CAD build for the part. Positions are in the model's coordinates, mm. Coordinates: 2 decimals unless noted, no trailing zeros. Loops run counter-clockwise (first coordinate to the right, second up) from the corner with the lowest first, then second, coordinate; pieces in that order, holes last. Notation, with made-up numbers: (4, -37.75) -> (10, -37.75) arc R17 cw to (10, -8.75) -> close; hole circle Ø7 at (35, -26). An arc over 180 degrees is marked (long way). Answer as a JSON object with one key per item and string values. Group by question number.
from build123d import *

# Parameters (mm, degrees)
SKETCH1_R           = 10
BOSS_EXTRUDE1_DEPTH = 60


with BuildPart() as part:
    # Sketch1 → Boss-Extrude1 (new body)
    with BuildSketch(Plane.XY):
        with BuildLine():
            Line((0, 0), (60, 0))
            Line((60, 0), (60, 60))
            ThreePointArc((60, 60), (30, 90), (0, 60))
            Line((0, 60), (0, 0))
        make_face()
        with Locations((30, 60)):
            Circle(SKETCH1_R, mode=Mode.SUBTRACT)
    extrude(amount=BOSS_EXTRUDE1_DEPTH)

    # Sketch4 → Cut-Revolve1 (revolve, cut)
    with BuildSketch(Plane.XY.offset(30)):
        with BuildLine():
            Line((30, 30), (30, -10))
            ThreePointArc((30, -10), (50, 10), (30, 30))
        make_face()
    revolve(axis=Axis((30, 30, 30), (0, -1, 0)), mode=Mode.SUBTRACT)


solid = part.part
Item 1: Band-saw the part on A-A, the plane z = 18. List the corners of the cut face in (x, y), and give its area (3 significant figures).
Item 2: Flat gauge pins, fed straight in: P1, Ø1, axis at y = 64.5, z = 48.5, coming from the -X side; P2, Ø2, axis at y = 64, z = 8.5, coming from the -X side. Where does each tip first touch, or does it go through?
Item 3: Pull direction Y, two halves, no side cores. Call faces 1 (the cylindrical face through (39.237, 56.17, 29.58)), 2 (the flat face through (30, 46, 60)), 3 (the cylindrical face through (30.66, 89.993, 29.58)): +Y half, -Y half, draft (parallel to the pull), parting line (faces both ways), or undercut.
Item 4: Drill centre lines: L1, parallel to Y at x = 30, z = 30; L2, parallel to X at y = 59.5, z = 5; L3, parallel to X at y = 66, z = 10. Where is each one in solid material? Low to high.
Item 5: Band-saw the part on C-C, the plane x = 30. List the corners of the cut face in (y, z).
Item 6: Band-saw the part on D-D, the plane y = 9. List the corners of the cut face in (x, z).
Item 7: Band-saw the part on B-B, the plane y = 55. List the corners of the cut face in (x, z).
Reply:
{
 "1": {"outline": "(0, 0) -> (17.51, 0) arc R16 cw (long way) to (42.49, 0) -> (60, 0) -> (60, 60) arc R30 ccw to (0, 60) -> close; hole circle Ø20 at (30, 60)", "area": "4,000 mm²"},
 "2": {"P1": "x = 0.27", "P2": "x = 0.15"},
 "3": {"face 1": "undercut", "face 2": "draft", "face 3": "+Y half"},
 "4": {"L1": "30 to 50, 70 to 90", "L2": "0 to 20.01, 39.99 to 60", "L3": "0.61 to 22, 38 to 59.39"},
 "5": {"outline": "(0, 0) -> (50, 0) -> (50, 60) -> (0, 60) -> (0, 47.32) arc R20 cw (long way) to (0, 12.68) -> close; (70, 0) -> (90, 0) -> (90, 60) -> (70, 60) -> close"},
 "6": {"outline": "(0, 0) -> (60, 0) -> (60, 60) -> (0, 60) -> close; hole circle Ø39.95 at (30, 30)"},
 "7": {"outline": "(0, 0) -> (21.34, 0) -> (21.34, 60) -> (0, 60) -> close; (38.66, 0) -> (60, 0) -> (60, 60) -> (38.66, 60) -> close"}
}
